```python
from build123d import *

# Parameters (mm, degrees)
F0_R     = 40
F1_DEPTH = 30
F2_DEPTH = 15
F3_DEPTH = 25


with BuildPart() as f1:
    # F0 (on Front) → F1 (new body, symmetric)
    with BuildSketch(Plane.XZ):
        with BuildLine():
            ThreePointArc((41.733687, -40.277778), (58.167604, -28.977662), (77.711003, -25))
            Line((77.711003, -25), (167.711003, -25))
            ThreePointArc((167.711003, -25), (191.531756, -7.587605), (182.1704, 20.39426))
            ThreePointArc((182.1704, 20.39426), (175.298608, 23.820752), (167.711003, 25))
            Line((167.711003, 25), (77.711003, 25))
            ThreePointArc((77.711003, 25), (58.167604, 28.977662), (41.733687, 40.277778))
            ThreePointArc((41.733687, 40.277778), (11.387237, 56.871177), (-23.008546, 53.241026))
            ThreePointArc((-23.008546, 53.241026), (-47.687518, -33.013643), (41.733687, -40.277778))
        make_face()
        Circle(F0_R, mode=Mode.SUBTRACT)
        with BuildLine():
            ThreePointArc((77.711003, -12.5), (65.211003, 0), (77.711003, 12.5))
            Line((77.711003, 12.5), (167.711003, 12.5))
            ThreePointArc((167.711003, 12.5), (180.211003, 0), (167.711003, -12.5))
            Line((167.711003, -12.5), (77.711003, -12.5))
        make_face(mode=Mode.SUBTRACT)
    extrude(amount=F1_DEPTH, both=True)

    # F0 (on Front) → F2 (join, symmetric)
    with BuildSketch(Plane.XZ):
        with BuildLine():
            ThreePointArc((-16.207991, 85.12381), (-11.382532, 67.427879), (-23.008546, 53.241026))
            ThreePointArc((-23.008546, 53.241026), (11.387237, 56.871177), (41.733687, 40.277778))
            ThreePointArc((41.733687, 40.277778), (58.167604, 28.977662), (77.711003, 25))
            Line((77.711003, 25), (167.711003, 25))
            ThreePointArc((167.711003, 25), (175.298608, 23.820752), (182.1704, 20.39426))
            Line((182.1704, 20.39426), (70.561858, 99.523988))
            ThreePointArc((70.561858, 99.523988), (78.694101, 93.226812), (86.267027, 86.267027))
            ThreePointArc((86.267027, 86.267027), (86.267027, 55.154329), (55.154329, 55.154329))
            ThreePointArc((55.154329, 55.154329), (29.849308, 72.062604), (0, 78))
            ThreePointArc((0, 78), (-8.852226, 79.859541), (-16.207991, 85.12381))
        make_face()
    extrude(amount=F2_DEPTH, both=True)

    # F0 (on Front) → F3 (join, symmetric)
    with BuildSketch(Plane.XZ):
        with BuildLine():
            ThreePointArc((0, 122), (-20.140459, 108.852226), (-16.207991, 85.12381))
            ThreePointArc((-16.207991, 85.12381), (-8.852226, 79.859541), (0, 78))
            ThreePointArc((0, 78), (29.849308, 72.062604), (55.154329, 55.154329))
            ThreePointArc((55.154329, 55.154329), (86.267027, 55.154329), (86.267027, 86.267027))
            ThreePointArc((86.267027, 86.267027), (78.694101, 93.226812), (70.561858, 99.523988))
            ThreePointArc((70.561858, 99.523988), (37.027513, 116.245272), (0, 122))
        make_face()
        with BuildLine():
            ThreePointArc((0, 91), (-9, 100), (0, 109))
            ThreePointArc((0, 109), (41.712494, 100.702869), (77.074639, 77.074639))
            ThreePointArc((77.074639, 77.074639), (77.074639, 64.346717), (64.346717, 64.346717))
            ThreePointArc((64.346717, 64.346717), (34.824192, 84.073037), (0, 91))
        make_face(mode=Mode.SUBTRACT)
    extrude(amount=F3_DEPTH, both=True)


solid = f1.part
```
Here's how the part is built. I have some questions about the finished solid (model axes, mm). A direction names the side the tool comes from. Give positions to 0.01 mm unless a question says otherwise; leave off trailing zeros. Write each loop counter-clockwise with the first axis right and the second up, starting at its lowest first coordinate (ties: lowest second). Pieces come first, ordered by that corner, then holes. Notation, with made-up numbers: (14.25, -14) -> (70.25, -14) arc R18 cw to (70.25, -5) -> close; hole circle Ø7 at (51.5, -39.5). An arc over 180 degrees is marked (long way). Use one line per item in the form item = value.
1) If I drill on L1, parallel to Z at x = 31, y = -3.5; L2, parallel to Z at x = 125.5, y = 20.5; L3, parallel to Y at x = 148, z = 35, over which ranges is the centre line in solid material (lowest first)? Write a range as [from, to].
Verdict:
L1 = [-49.02, -25.28], [25.28, 85.56], [104.5, 118]
L2 = [-25, -12.5], [12.5, 25]
L3 = [-15, 15]
2) Suppose I cut it at D-D (z = 71.5). Please give me the cut outline in (x, y), and give its area (3 significant figures).
Verdict:
outline = (-10.94, -15) -> (31.17, -15) -> (31.17, -25) -> (56.29, -25) -> (56.29, 25) -> (31.17, 25) -> (31.17, 15) -> (-10.94, 15) -> close; (79.68, -25) -> (92.7, -25) -> (92.7, -15) -> (110.09, -15) -> (110.09, 15) -> (92.7, 15) -> (92.7, 25) -> (79.68, 25) -> close
area = 3,690 mm2
3) Suppose I cut it at C-C (x = 135). Please give me the cut outline in (y, z), and give its area (3 significant figures).
Verdict:
outline = (-30, -25) -> (30, -25) -> (30, -12.5) -> (-30, -12.5) -> close; (-30, 12.5) -> (30, 12.5) -> (30, 25) -> (15, 25) -> (15, 53.84) -> (-15, 53.84) -> (-15, 25) -> (-30, 25) -> close
area = 2,370 mm2
4) I'm going to push flat-ended pins straight in: pin 1 (12 mm diameter, centred on x = 122, y = -20, fed in from +Z); pin 2 (5 mm diameter, centred on x = 9, y = 15, fed in from -Z); pin 3 (12 mm diameter, centred on x = 136, y = 26, fed in from +Z); pin 4 (10 mm diameter, centred on x = 100, z = 28, fed in from -Y). Where does each tip first touch, or does it pass through?
Verdict:
pin_1 = 65.41
pin_2 = -57.63
pin_3 = 25
pin_4 = -30
5) We'd pull the mould along X, two halves only. Please class faces 4 (the face through (-11.33, -0.21, 67.69)), 5 (the face through (85.921, 19.93, 54.816)), 6 (the face through (78.804, -20.07, 93.134)): +X half, -X half, draft (parallel to the pull), parting line (faces both ways), or undercut.
Verdict:
face_4 = -X half
face_5 = undercut
face_6 = +X half
6) Suppose I cut it at A-A (z = 0). Please give me the cut outline in (x, y), and give its area (3 significant figures).
Verdict:
outline = (-58, -30) -> (-40, -30) -> (-40, 30) -> (-58, 30) -> close; (40, -30) -> (65.21, -30) -> (65.21, 30) -> (40, 30) -> close; (180.21, -30) -> (192.71, -30) -> (192.71, 30) -> (180.21, 30) -> close
area = 3,340 mm2
7) On a 3-axis mill with a long thin cutter (end or side, diameter ignored), from which of +Z, -Z, +X, -X, +Y, -Y can I reach the whole of each face in a straight line? I mean faces 1 (the face through (58.427, 22.395, 28.869)), 2 (the face through (78.804, 19.93, 93.134)), 3 (the face through (79, -15, 45)). Say none if no direction works.
Verdict:
face_1 = +X, +Y
face_2 = +Z, +X, +Y
face_3 = -Y
8) Suppose I cut it at B-B (y = 12). Please give me the cut outline in (x, z), and give its area (3 significant figures).
Verdict:
outline = (-23.01, 53.24) arc R58 ccw (long way) to (41.73, -40.28) arc R50 cw to (77.71, -25) -> (167.71, -25) arc R25 ccw to (182.17, 20.39) -> (70.56, 99.52) arc R122 ccw to (0, 122) arc R22 ccw to (-16.21, 85.12) arc R20 cw to start; hole circle Ø80 at (0, 0); hole (0, 91) arc R91 cw to (64.35, 64.35) arc R9 ccw to (77.07, 77.07) arc R109 ccw to (0, 109) arc R9 ccw to start; hole (77.71, -12.5) -> (167.71, -12.5) arc R12.5 ccw to (167.71, 12.5) -> (77.71, 12.5) arc R12.5 ccw to start
area = 17,800 mm2
